Geometry: see drawing. Coordinates: mm, zero at the bounding-box minimum. Coordinates: 2 decimals unless noted, no trailing zeros. Loops run counter-clockwise (first coordinate to the right, second up) from the corner with the lowest first, then second, coordinate; pieces in that order, holes last. Notation, with made-up numbers: (12, 63.5) -> (22, 63.5) arc R27 cw to (22, 91.5) -> close; hole circle Ø8 at (-9, -17.75). An arc over 180 degrees is marked (long way). One line per question, with ' | ' between items. Start each with the question number.
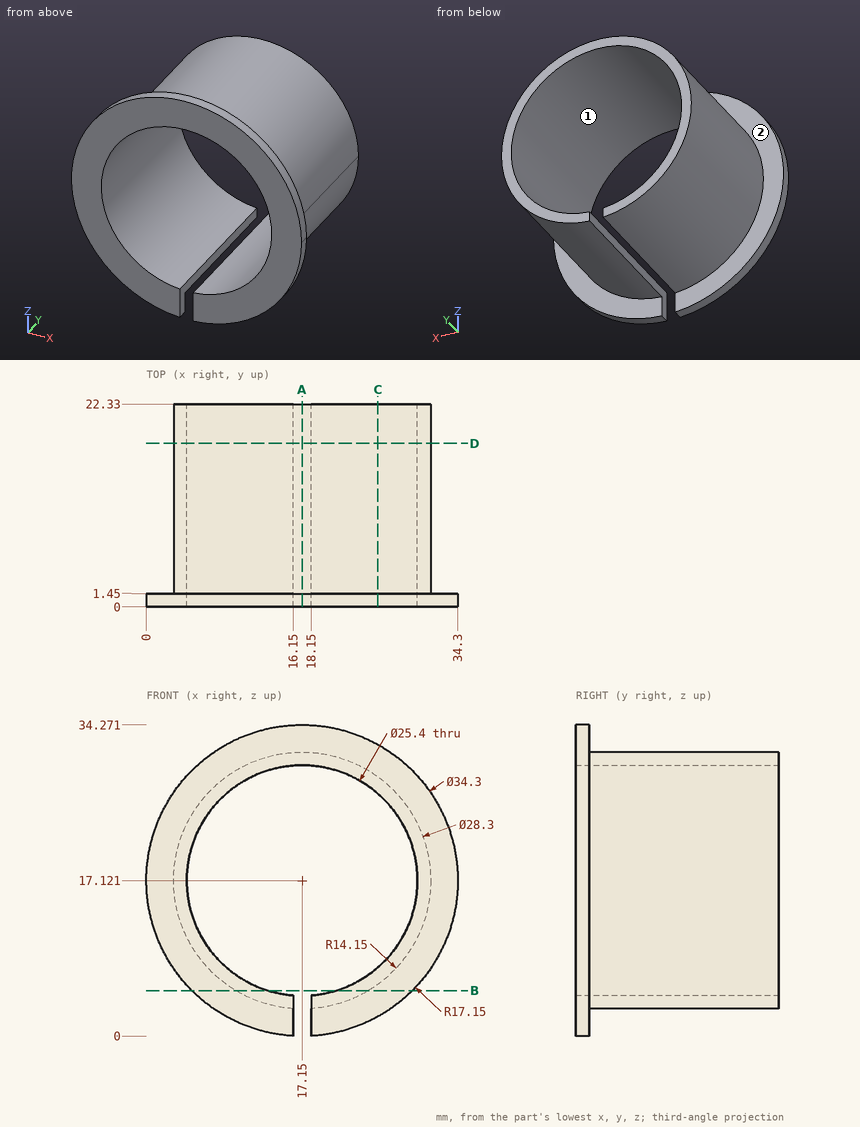
(1) Cut plane D-D, the plane y = 18. Return the cut outline in (x, z).
(2) Draft query along X for the marked faces 1 and 2. Return one class per face: pulls with the +X half, pulls with the -X half, needs draft (parallel to the pull), parting line crosses it, or undercut.
(3) Cut plane B-B, the plane z = 5. Return the cut outline in (x, y).
(4) Cut plane C-C, the plane x = 25.5. Return the cut outline in (y, z).
(5) Cut plane A-A, the plane x = 17.15. Return the cut outline in (y, z), and give its area (3 significant figures).
(6) Ray query, L1, parallel to Y at x = 28.5, z = 8; L2, parallel to Z at x = 17.15, y = 13; L3, parallel to X at y = 17.25, z = 16. Return the intervals inside material, ascending.
(7) Contact query for flat-ended pins moving along their axis: pin 1 Ø5 at (x, y) = (24.5, 7.5) entering from +Z; pin 2 Ø6 at (x, z) = (7, 28) entering from -Y; pin 3 Ø5 at (y, z) = (8, 1.5) entering from -X; pin 4 Ø5 at (x, y) = (26, 12.5) entering from -Z. Output: stop coordinate, or through.
Here are the results:
1) outline: (16.15, 3.01) -> (16.15, 4.46) arc R12.7 cw (long way) to (18.15, 4.46) -> (18.15, 3.01) arc R14.15 ccw (long way) to start
2) face 1: undercut | face 2: needs draft
3) outline: (5.02, 0) -> (13.36, 0) -> (13.36, 22.33) -> (9.85, 22.33) -> (9.85, 1.45) -> (5.02, 1.45) -> close; (20.94, 0) -> (29.28, 0) -> (29.28, 1.45) -> (24.45, 1.45) -> (24.45, 22.33) -> (20.94, 22.33) -> close
4) outline: (0, 2.14) -> (1.45, 2.14) -> (1.45, 5.7) -> (22.33, 5.7) -> (22.33, 7.55) -> (0, 7.55) -> close; (0, 26.69) -> (22.33, 26.69) -> (22.33, 28.54) -> (1.45, 28.54) -> (1.45, 32.1) -> (0, 32.1) -> close
5) outline: (0, 29.82) -> (22.33, 29.82) -> (22.33, 31.27) -> (1.45, 31.27) -> (1.45, 34.27) -> (0, 34.27) -> close | area: 36.7 mm2
6) L1: y = 0 to 1.45 | L2: z = 29.82 to 31.27 | L3: x = 3.04 to 4.5, 29.8 to 31.26
7) pin 1: stops at z = 30.41 | pin 2: stops at y = 0 | pin 3: stops at x = 11.85 | pin 4: stops at z = 4.48
